Verification items for the finished model (mm, model axes). Round coordinates to 2 decimals unless told otherwise and drop trailing zeros. Order: outer loops, then holes, each group sorted by start corner. A loop starts at its lowest first (then second) coordinate and runs counter-clockwise, first axis right, second up. Notation, with made-up numbers: (37, 85) -> (85, 85) arc R14 cw to (85, 93) -> close; hole circle Ø2 at (48.25, 83). An arc over 180 degrees is marked (long way). Return JSON: item names as keys, results as strings. Group by question number.
Item 1: Sectioned sample at C-C on y = 5.25. Record the cut outline in (x, z), plus the area to 3 significant figures.
Item 2: Sectioned sample at D-D on x = -48. Record the cut outline in (y, z).
Item 3: Sectioned sample at B-B on x = 3. Record the cut outline in (y, z).
Item 4: Depth check by flat-ended pin: pin 1 Ø1.5 at (y, z) = (1.5, 28.5) entering from -X; pin 2 Ø3 at (y, z) = (3, 21.5) entering from +X; pin 3 Ø1.5 at (x, y) = (13.5, 4) entering from +Z. Enter the tip coordinate at first touch or a pass-through.
Item 5: Sectioned sample at A-A on z = 0. Record the cut outline in (x, y).
Item 6: Scan lines: probe 1 along Z at (x, y) = (0, 2.5); probe 2 along Z at (x, y) = (-2.5, 1.5); probe 3 along X at (y, z) = (4, 0). Record each from-to range of solid material in increasing order. Write a range as from..to.
Item 7: Draft check along X on faces 1 (the flat face through (27, 6.35, 13)), 2 (the cylindrical face through (-0.8, 3.1, -57.1)), 3 (the cylindrical face through (-13.77, 3.13, 61.99)). Enter one of: pulls with the +X half, pulls with the -X half, needs draft (parallel to the pull), parting line crosses it, or undercut.
```python
from build123d import *

# Parameters (mm, degrees)
SKETCH1_R           = 63.5
SKETCH1_R_2         = 29.083
SKETCH1_R_3         = 6.35
BOSS_EXTRUDE1_DEPTH = 6.35
SKETCH5_R           = 3.302
CUT_EXTRUDE4_DEPTH  = 7.35
CIRPATTERN2_COUNT   = 3


with BuildPart() as part:
    # Sketch1 → Boss-Extrude1 (new body)
    with BuildSketch(Plane(origin=(0, 0, 0), x_dir=(1, 0, 0), z_dir=(0, 1, 0))):
        Circle(SKETCH1_R)
        Circle(SKETCH1_R_2, mode=Mode.SUBTRACT)
        with Locations((0, 50.8)):
            Circle(SKETCH1_R_3, mode=Mode.SUBTRACT)
        with Locations((43.994090512, -25.4)):
            Circle(SKETCH1_R_3, mode=Mode.SUBTRACT)
        with Locations((-43.994090512, -25.4)):
            Circle(SKETCH1_R_3, mode=Mode.SUBTRACT)
    extrude(amount=BOSS_EXTRUDE1_DEPTH)

    # Sketch5 → Cut-Extrude4 (cut, through all)
    with BuildSketch(Plane(origin=(0, 6.35, 0), x_dir=(1, 0, 0), z_dir=(0, 1, 0))):
        with Locations((-43.229109276, 14.884976022)):
            Circle(SKETCH5_R)
    cut_extrude4 = extrude(amount=-CUT_EXTRUDE4_DEPTH, mode=Mode.SUBTRACT)

    # CirPattern2: Cut-Extrude4 ×3 about axis
    cirpattern2_axis = Axis((0, 0, 0), (0, 1, 0))
    for i in range(1, CIRPATTERN2_COUNT):
        add(cut_extrude4.rotate(cirpattern2_axis, i * 360 / CIRPATTERN2_COUNT), mode=Mode.SUBTRACT)


solid = part.part
```
Recorded:
{
 "1": {"outline": "circle Ø127 at (0, 0); hole circle Ø12.7 at (-43.99, 25.4); hole circle Ø6.6 at (-43.23, -14.88); hole circle Ø58.17 at (0, 0); hole circle Ø12.7 at (0, -50.8); hole circle Ø6.6 at (8.72, 44.88); hole circle Ø6.6 at (34.51, -30); hole circle Ø12.7 at (43.99, 25.4)", "area": "9,530 mm²"},
 "2": {"outline": "(0, -41.57) -> (6.35, -41.57) -> (6.35, 20.47) -> (0, 20.47) -> close; (0, 30.33) -> (6.35, 30.33) -> (6.35, 41.57) -> (0, 41.57) -> close"},
 "3": {"outline": "(0, -63.43) -> (6.35, -63.43) -> (6.35, -56.4) -> (0, -56.4) -> close; (0, -45.2) -> (6.35, -45.2) -> (6.35, -28.93) -> (0, -28.93) -> close; (0, 28.93) -> (6.35, 28.93) -> (6.35, 63.43) -> (0, 63.43) -> close"},
 "4": {"pin 1": "x = -57.12", "pin 2": "x = 60.27", "pin 3": "z = 62.21"},
 "5": {"outline": "(-63.5, 0) -> (-29.08, 0) -> (-29.08, 6.35) -> (-63.5, 6.35) -> close; (29.08, 0) -> (63.5, 0) -> (63.5, 6.35) -> (29.08, 6.35) -> close"},
 "6": {"probe 1": "-63.5..-57.15, -44.45..-29.08, 29.08..63.5", "probe 2": "-63.45..-56.64, -44.96..-28.98, 28.98..63.45", "probe 3": "-63.5..-29.08, 29.08..63.5"},
 "7": {"face 1": "needs draft", "face 2": "undercut", "face 3": "parting line crosses it"}
}
